Verification items for this drawing (mm, ordinates from the low corner). Round coordinates to 2 decimals unless told otherwise and drop trailing zeros. Loops run counter-clockwise (first coordinate to the right, second up) from the corner with the lowest first, then second, coordinate; pieces in that order, holes last. Notation, with made-up numbers: (-38.5, 57) - (0.5, 57) arc R18 ccw to (0.5, 63) - close; hole circle Ø3 at (30, 37.5). An arc over 180 degrees is marked (long way). Put each result on its own line as item: value. Start each with the question number.
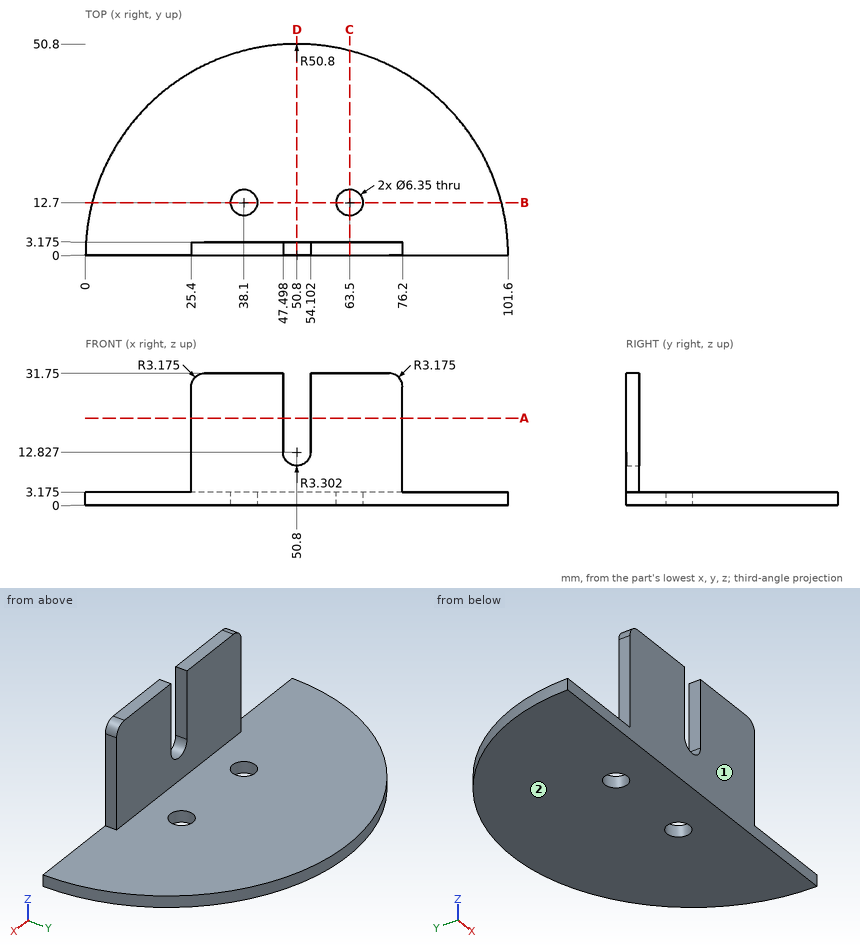
Q1. Cross-section at A-A on z = 21. Enter the section's corners in (x, y) (3 decimals).
Q2. Depth check by flat-ended pin: pin 1 Ø1 at (y, z) = (1.5, 17) entering from +X; pin 2 Ø1 at (x, z) = (66, 16.5) entering from +Y (3 decimals); pin 3 Ø1 at (x, y) = (74.5, 9.5) entering from +Z (3 decimals); pin 4 Ø3 at (y, z) = (45, 6) entering from -X. Enter the tip coordinate at first touch or a pass-through.
Q3. Cross-section at C-C on x = 63.5. Enter the section's corners in (y, z) (3 decimals), and give its area (3 significant figures).
Q4. Cross-section at B-B on y = 12.7. Enter the section's corners in (x, z) (3 decimals), and give its area (3 significant figures).
Q5. Material ranges on line 1 (X direction, y = 12, z = 1); line 2 (Z direction, x = 33.5, y = 9.5) (3 decimals), recorded low to high. Write a range as from..to.
Q6. Cross-section at D-D on x = 50.8. Enter the section's corners in (y, z) (3 decimals).
Q7. Draft check along Z on the marked faces 1 and 2. Enter one of: +Z half, -Z half, draft (parallel to the pull), parting line (faces both ways), or undercut.
Answer list:
1. outline: (25.4, 0) - (47.498, 0) - (47.498, 3.175) - (25.4, 3.175) - close; (54.102, 0) - (76.2, 0) - (76.2, 3.175) - (54.102, 3.175) - close
2. pin 1: stops at x = 76.2
2. pin 2: stops at y = 3.175
2. pin 3: stops at z = 3.175
2. pin 4: passes through
3. outline: (0, 0) - (9.525, 0) - (9.525, 3.175) - (3.175, 3.175) - (3.175, 31.75) - (0, 31.75) - close; (15.875, 0) - (49.187, 0) - (49.187, 3.175) - (15.875, 3.175) - close
3. area: 227 mm2
4. outline: (1.613, 0) - (34.925, 0) - (34.925, 3.175) - (1.613, 3.175) - close; (41.275, 0) - (60.325, 0) - (60.325, 3.175) - (41.275, 3.175) - close; (66.675, 0) - (99.987, 0) - (99.987, 3.175) - (66.675, 3.175) - close
4. area: 272 mm2
5. line 1: x = 1.44..35, 41.2..60.4, 66.6..100.16
5. line 2: z = 0..3.175
6. outline: (0, 0) - (50.8, 0) - (50.8, 3.175) - (3.175, 3.175) - (3.175, 9.525) - (0, 9.525) - close
7. face 1: draft
7. face 2: -Z half
